Check sheet for the modelled part. Datum: model origin and axes. Units: mm. A direction names the side the tool comes from. Round coordinates to 2 decimals unless told otherwise and drop trailing zeros. Loops run counter-clockwise (first coordinate to the right, second up) from the corner with the lowest first, then second, coordinate; pieces in that order, holes last. Notation, with made-up numbers: (0.5, 0.5) - (30.5, 0.5) arc R29 cw to (30.5, 20.5) - close; hole circle Ø7 at (19.5, -3). An arc over 180 degrees is marked (long way). Put each result on its own line as item: value. Start each with the question number.
Item 1: Section check B-B, the plane z = 52. Record the cut outline in (x, y).
Item 2: Material ranges on line 1 along Z through (x, y) = (33, -36); line 2 along X through (y, z) = (-16.5, 86.5); line 3 along Z through (x, y) = (7.5, -41), recorded low to high.
Item 3: Section check C-C, the plane x = 43.5. Record the cut outline in (y, z).
Item 4: Gauge pin test, flat ends, axial feed: pin 1 Ø4 at (y, z) = (1, 51) entering from +X; pin 2 Ø12 at (y, z) = (-3.5, 79) entering from +X; pin 3 Ø8 at (x, y) = (7, -38) entering from +Z. Record the tip position at first contact, or that the pin passes through.
Item 5: Tool access check on faces 1 (the flat face through (-12, 50, 38)), 2 (the flat face through (-16, -1, 83)). Record the directions out of +Z, -Z, +X, -X, +Y, -Y that give a thin tool (end or side, any length) a straight path to the whole face; none if there is none.
Item 6: Section check A-A, the plane y = -8. Record the cut outline in (x, z).
from build123d import *

# Parameters (mm, degrees)
F0_W     = 100
F0_H     = 100
F1_DEPTH = 100
F3_DEPTH = 100


with BuildPart() as f1:
    # F0 (on Top) → F1 (new body)
    with BuildSketch(Plane.XY):
        Rectangle(F0_W, F0_H)
    extrude(amount=F1_DEPTH)

    # F2 (on face) → F3 (cut)
    with BuildSketch(Plane.XZ.offset(50)):
        Polygon((50, 100), (-16, 100), (-16, 64.911917), (17, 64.911917), (17, 38.397651), (50, 38.397651), align=None)
    extrude(amount=-F3_DEPTH, mode=Mode.SUBTRACT)


solid = f1.part
Check result:
1. outline: (-50, -50) - (17, -50) - (17, 50) - (-50, 50) - close
2. line 1: 0 to 38.4
2. line 2: -50 to -16
2. line 3: 0 to 64.91
3. outline: (-50, 0) - (50, 0) - (50, 38.4) - (-50, 38.4) - close
4. pin 1: x = 17
4. pin 2: x = -16
4. pin 3: z = 64.91
5. face 1: +Z, -Z, +X, -X, +Y
5. face 2: +Z, +X, +Y, -Y
6. outline: (-50, 0) - (50, 0) - (50, 38.4) - (17, 38.4) - (17, 64.91) - (-16, 64.91) - (-16, 100) - (-50, 100) - close
